Check sheet for the modelled part. Datum: model origin and axes. Units: mm. Face numbers are marked on the shaded views. A direction names the side the tool comes from. Round coordinates to 2 decimals unless told otherwise and drop trailing zeros. Write each loop counter-clockwise with the first axis right and the second up, starting at its lowest first coordinate (ties: lowest second). Pieces come first, ordered by that corner, then holes. Notation, with made-up numbers: (65.5, 83.5) -> (110.5, 83.5) arc R10 cw to (110.5, 87.5) -> close; hole circle Ø10 at (35.25, -4.5). An arc over 180 degrees is marked (long way). One line per item, written item: value.
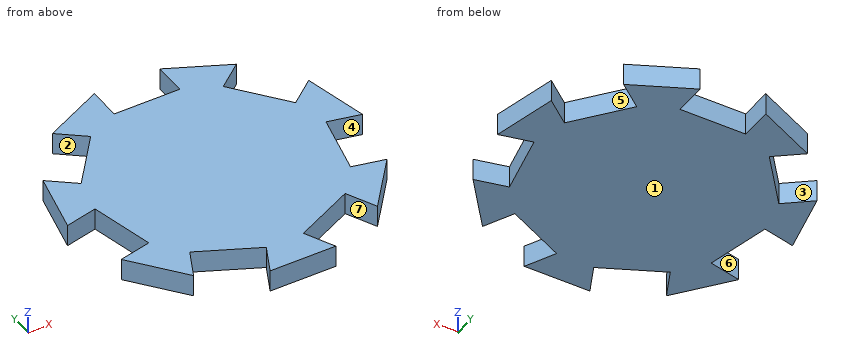
from build123d import *

# Parameters (mm, degrees)
F1_DEPTH = 2.116667


with BuildPart() as f1:
    # F0 (on Top) → F1 (new body, symmetric)
    with BuildSketch(Plane.XY):
        Polygon((-6.35, 21.471168), (-6.35, 27.821168), (-17.792305, 22.310844), (-12.827675, 18.351684), (-20.745995, 8.422424), (-25.710625, 12.381584), (-28.536641, 0), (-22.345849, 1.413008), (-19.519833, -10.968577), (-25.710625, -12.381584), (-17.792305, -22.310844), (-15.037143, -16.589692), (-3.594838, -22.100015), (-6.35, -27.821168), (6.35, -27.821168), (3.594838, -22.100015), (15.037143, -16.589692), (17.792305, -22.310844), (25.710625, -12.381584), (19.519833, -10.968577), (22.345849, 1.413008), (28.536641, 0), (25.710625, 12.381584), (20.745995, 8.422424), (12.827675, 18.351684), (17.792305, 22.310844), (6.35, 27.821168), (6.35, 21.471168), align=None)
    extrude(amount=F1_DEPTH, both=True)


solid = f1.part
Item 1: Thickness scan on line 1 (X direction, y = -18, z = 0.75); line 2 (X direction, y = -22, z = -1.05); line 3 (Y direction, x = 15.5, z = 1.2). Record the ranges inside material, lowest first.
Answer:
line 1: x = -21.23 to -15.72, -12.11 to 12.11, 15.72 to 21.23
line 2: x = -18.04 to -17.64, -3.8 to 3.8, 17.64 to 18.04
line 3: y = -17.55 to 15, 20.48 to 23.41
Item 2: Mould release check, pull along X, two halves, no side actions. Record for the marked faces 1, 2, 3 and 4: pulls with the +X half, pulls with the -X half, needs draft (parallel to the pull), parting line crosses it, or undercut.
Answer:
face 1: needs draft
face 2: pulls with the -X half
face 3: undercut
face 4: undercut
Item 3: Sectioned sample at A-A on z = 1.35. Enter the section's corners in (x, y), and give its area (3 significant figures).
Answer:
outline: (-28.54, 0) -> (-22.35, 1.41) -> (-19.52, -10.97) -> (-25.71, -12.38) -> (-17.79, -22.31) -> (-15.04, -16.59) -> (-3.59, -22.1) -> (-6.35, -27.82) -> (6.35, -27.82) -> (3.59, -22.1) -> (15.04, -16.59) -> (17.79, -22.31) -> (25.71, -12.38) -> (19.52, -10.97) -> (22.35, 1.41) -> (28.54, 0) -> (25.71, 12.38) -> (20.75, 8.42) -> (12.83, 18.35) -> (17.79, 22.31) -> (6.35, 27.82) -> (6.35, 21.47) -> (-6.35, 21.47) -> (-6.35, 27.82) -> (-17.79, 22.31) -> (-12.83, 18.35) -> (-20.75, 8.42) -> (-25.71, 12.38) -> close
area: 1,910 mm^2
Item 4: Sectioned sample at C-C on x = 2. Enter the section's corners in (y, z), and give its area (3 significant figures).
Answer:
outline: (-27.82, -2.12) -> (21.47, -2.12) -> (21.47, 2.12) -> (-27.82, 2.12) -> close
area: 209 mm^2
Item 5: Tool access check on the marked faces 5, 6 and 7. Record the directions out of +Z, -Z, +X, -X, +Y, -Y that give a thin tool (end or side, any length) a straight path to the whole face; none if there is none.
Answer:
face 5: +Z, -Z
face 6: +Z, -Z, -X
face 7: +Z, -Z, -Y
Item 6: Depth check by flat-ended pin: P1, Ø1, axis at y = -7.5, z = -0.5, coming from the +X side; P2, Ø1.3, axis at y = 24, z = 0, coming from the -X side; P3, Ø2, axis at x = 0.5, z = 1, coming from the +Y side. Enter the tip coordinate at first touch or a pass-through.
Answer:
P1: stops at x = 20.43
P2: stops at x = -15.63
P3: stops at y = 21.47
Item 7: Sectioned sample at B-B on x = 24. Enter the section's corners in (y, z).
Answer:
outline: (-14.53, -2.12) -> (-11.99, -2.12) -> (-11.99, 2.12) -> (-14.53, 2.12) -> close; (1.04, -2.12) -> (11.02, -2.12) -> (11.02, 2.12) -> (1.04, 2.12) -> close
Item 8: Sectioned sample at D-D on y = 4. Enter the section's corners in (x, z), and give its area (3 significant figures).
Answer:
outline: (-27.62, -2.12) -> (27.62, -2.12) -> (27.62, 2.12) -> (-27.62, 2.12) -> close
area: 234 mm^2
